Could you check a few things on this model? Use its own coordinates, in mm. A direction names the side the tool comes from. Coordinates: 2 decimals unless noted, no trailing zeros. Loops run counter-clockwise (first coordinate to the right, second up) from the corner with the lowest first, then second, coordinate; pieces in that order, holes last. Notation, with made-up numbers: (35, 89.5) -> (56, 89.5) arc R27 ccw to (56, 106.5) -> close; hole circle Ø8 at (45.25, 63.25). An arc over 180 degrees is marked (long way). One line per question, with ' | ' between items.
```python
from build123d import *

# Parameters (mm, degrees)
SKETCH1_W           = 29.9974
SKETCH1_H           = 19.6342
BOSS_EXTRUDE1_DEPTH = 1.4859
SKETCH2_W           = 19.610793651
SKETCH2_H           = 8.55658582
BOSS_EXTRUDE2_DEPTH = 1.4859
SKETCH3_W           = 19.6342
SKETCH3_H           = 8.73321644
BOSS_EXTRUDE3_DEPTH = 1.4859


with BuildPart() as part:
    # Sketch1 → Boss-Extrude1 (new body)
    with BuildSketch(Plane(origin=(0, 0, 0), x_dir=(1, 0, 0), z_dir=(0, 1, 0))):
        Rectangle(SKETCH1_W, SKETCH1_H)
    extrude(amount=BOSS_EXTRUDE1_DEPTH)

    # Sketch2 → Boss-Extrude2 (add)
    with BuildSketch(Plane(origin=(-14.9987, 0, 0), x_dir=(0, 0, -1), z_dir=(1, 0, 0))):
        with Locations((-0.011703175, 4.27829291)):
            Rectangle(SKETCH2_W, SKETCH2_H)
    extrude(amount=-BOSS_EXTRUDE2_DEPTH)

    # Sketch3 → Boss-Extrude3 (add)
    with BuildSketch(Plane(origin=(14.9987, 0, 0), x_dir=(0, 0, -1), z_dir=(1, 0, 0))):
        with Locations((0, 4.36660822)):
            Rectangle(SKETCH3_W, SKETCH3_H)
    extrude(amount=BOSS_EXTRUDE3_DEPTH)


solid = part.part
```
Q1. For faces 1 (the face through (-16, 8.557, 0)), 2 (the face through (0, 1.486, 0)), 3 (the face through (16, 8.733, 0)), which set-ups out of +Z, -Z, +X, -X, +Y, -Y let a thin tool reach every point of the face, with its end or its side?
Values follow:
face 1: +Z, -Z, -X, +Y | face 2: +Z, -Z, +Y | face 3: +Z, -Z, +X, -X, +Y
Q2. We'd pull the mould along X, two halves only. Please class faces 4 (the face through (16.485, 4, 0)), 5 (the face through (-14.999, 5, 0)), 6 (the face through (-16.485, 4, 0)), 7 (the face through (-16, 4, -9.794)): released by +X, released by -X, zero draft, split by the parting line, or undercut.
Values follow:
face 4: released by +X | face 5: undercut | face 6: released by -X | face 7: zero draft
Q3. For pin 1 (4 mm diameter, centred on x = -8.5, z = -5, fed in from +Y); pin 2 (1.2 mm diameter, centred on x = -16, y = 4.5, fed in from -Z), each with a flat end and sliding along its axis, tell me the tip position at first contact or that it passes through.
Values follow:
pin 1: stops at y = 1.49 | pin 2: stops at z = -9.79
Q4. Imagine slicing it at A-A on y = 2. Write out the boundary of the cut face in (x, z), plus the area to 3 significant figures.
Values follow:
outline: (-16.48, -9.79) -> (-15, -9.79) -> (-15, 9.82) -> (-16.48, 9.82) -> close; (15, -9.82) -> (16.48, -9.82) -> (16.48, 9.82) -> (15, 9.82) -> close | area: 58.3 mm2
Q5. Imagine slicing it at C-C on x = -8. Write out the boundary of the cut face in (y, z).
Values follow:
outline: (0, -9.82) -> (1.49, -9.82) -> (1.49, 9.82) -> (0, 9.82) -> close
Q6. Imagine slicing it at B-B on z = -5.5. Write out the boundary of the cut face in (x, y).
Values follow:
outline: (-16.48, 0) -> (16.48, 0) -> (16.48, 8.73) -> (15, 8.73) -> (15, 1.49) -> (-15, 1.49) -> (-15, 8.56) -> (-16.48, 8.56) -> close
Q7. Please list where these lines run through material, in increasing order: L1, parallel to X at y = 8.25, z = 8.5; L2, parallel to Y at x = 11, z = 5.5. Write a range as [from, to].
Values follow:
L1: x = [-16.48, -15], [15, 16.48] | L2: y = [0, 1.49]
